The listing builds one solid part. Answer for the finished solid, in the listing's coordinates (mm). Face numbers are marked on the shaded views. A direction names the side the tool comes from. Give positions to 0.01 mm unless a question says otherwise; leave off trailing zeros. Order: outer loops, then holes, each group sorted by start corner. A loop starts at its lowest first (then second) coordinate and runs counter-clockwise, first axis right, second up. Notation, with made-up numbers: (88, -10.75) - (142, -10.75) arc R26 ccw to (142, 19.25) - close; hole circle Ø10 at (51, 22). An arc over 180 degrees is marked (long way). Answer in a Markdown table with one row per item. Add a question column.
```python
from build123d import *

# Parameters (mm, degrees)
PAD027_DEPTH    = 40
PAD028_DEPTH    = 52.4
SKETCH048_W     = 90.6
SKETCH048_H     = 42.3
PAD029_DEPTH    = 1
SKETCH049_R     = 38
POCKET015_DEPTH = 1
POCKET016_DEPTH = 46.3
SKETCH051_R     = 2.15
POCKET017_DEPTH = 1
SKETCH063_W     = 90.6
SKETCH063_H     = 1
PAD033_DEPTH    = 18
SKETCH069_R     = 3.25
POCKET028_DEPTH = 1
SKETCH071_W     = 4
SKETCH071_H     = 6
POCKET030_DEPTH = 1


with BuildPart() as part:
    # Sketch047 → Pad027 (new body)
    with BuildSketch(Plane.XZ):
        Polygon((-45.3, 42), (-46.3, 42), (-46.3, 85.3), (46.3, 85.3), (46.3, 42), (45.3, 42), (45.3, 84.3), (-45.3, 84.3), align=None)
    extrude(amount=PAD027_DEPTH)

    # Sketch047 → Pad028 (join)
    with BuildSketch(Plane.XZ):
        Polygon((-45.3, 42), (-46.3, 42), (-46.3, 85.3), (46.3, 85.3), (46.3, 42), (45.3, 42), (45.3, 84.3), (-45.3, 84.3), align=None)
    extrude(amount=-PAD028_DEPTH)

    # Sketch048 → Pad029 (join)
    with BuildSketch(Plane.XZ):
        with Locations((0, 63.15)):
            Rectangle(SKETCH048_W, SKETCH048_H)
    extrude(amount=PAD029_DEPTH)

    # Sketch049 → Pocket015 (cut)
    with BuildSketch(Plane.XZ):
        with Locations((0, 43)):
            Circle(SKETCH049_R)
    extrude(amount=POCKET015_DEPTH, mode=Mode.SUBTRACT)

    # Sketch050 → Pocket016 (cut, symmetric)
    with BuildSketch(Plane.YZ):
        Polygon((-5, 42), (-40, 84.3), (-40, 42), align=None)
    extrude(amount=POCKET016_DEPTH, both=True, mode=Mode.SUBTRACT)

    # Sketch051 → Pocket017 (cut)
    with BuildSketch(Plane.XZ):
        with Locations((-35.75, 78.75)):
            Circle(SKETCH051_R)
        with Locations((35.75, 78.75)):
            Circle(SKETCH051_R)
    extrude(amount=POCKET017_DEPTH, mode=Mode.SUBTRACT)

    # Sketch063 (on Face12 of Pocket017) → Pad033 (join)
    with BuildSketch(Plane(origin=(0, 0, 84.3), x_dir=(1, 0, 0), z_dir=(0, 0, -1))):
        with Locations((0, 22.5)):
            Rectangle(SKETCH063_W, SKETCH063_H)
    extrude(amount=PAD033_DEPTH)

    # Sketch069 (on Face13 of Pad033) → Pocket028 (cut)
    with BuildSketch(Plane.XZ.offset(23)):
        with Locations((-35.75, 78.75)):
            Circle(SKETCH069_R)
        with Locations((35.75, 78.75)):
            Circle(SKETCH069_R)
    extrude(amount=-POCKET028_DEPTH, mode=Mode.SUBTRACT)

    # Sketch071 → Pocket030 (cut)
    with BuildSketch(Plane.XZ):
        with Locations((43.3, 81.3)):
            Rectangle(SKETCH071_W, SKETCH071_H)
    extrude(amount=POCKET030_DEPTH, mode=Mode.SUBTRACT)


solid = part.part
```
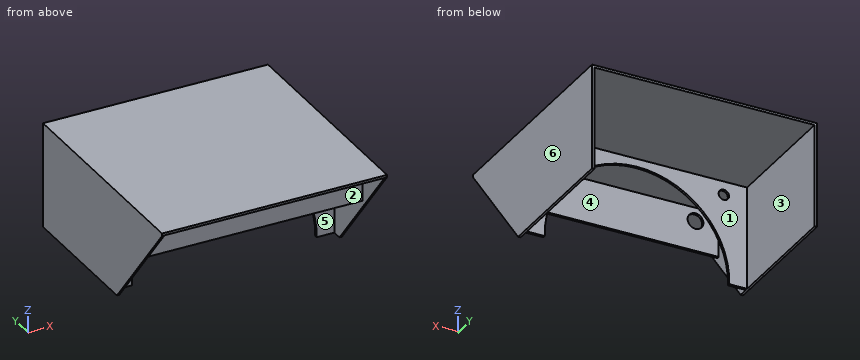
(1) For the marked faces 5 and 6, determine the directions among +Z, -Z, +X, -X, +Y, -Y from which every point of the face is accessible in a straight line to the end or side of a thin tool.
(2) Find section A-A, the plane x = 0. Write down the section's boundary in (y, z), plus the area to 3 significant figures.
(3) Find section B-B, the plane z = 46. Write down the section's boundary in (x, y).
(4) The mould has two halves that part along Y. Classify the marked faces 1, 2, 3 and 4: +Y half, -Y half, draft (parallel to the pull), parting line (faces both ways), or undercut.
(5) Each of these flat-tipped pins is pushed along its axis until it touches: P1, Ø22.5, axis at x = -6, y = 2, coming from the -Z side; P2, Ø12.5, axis at x = 11.5, z = 61, coming from the -Y side; P3, Ø0.5, axis at x = 22, y = -22.5, coming from the -Z side. Where does it stop, or does it pass through?
(6) Find section C-C, the plane x = 35.75. Write down the section's boundary in (y, z), plus the area to 3 significant figures.
(7) Find section D-D, the plane y = 37.5. Write down the section's boundary in (x, z).
(8) Straight lines are drawn through the part: line 1 (Y direction, x = 10, z = 83.5); line 2 (X direction, y = 21, z = 66.5); line 3 (Z direction, x = -35.75, y = -22.75). For each, find the intervals that lie inside material, in ascending order.
Answer key:
| question | item | result |
|---|---|---|
| 1 | face 5 | -Z |
| 1 | face 6 | +Z, -Z, +X, +Y, -Y |
| 2 | outline | (-40, 84.3) - (-23, 84.3) - (-23, 66.3) - (-22, 66.3) - (-22, 84.3) - (-1, 84.3) - (-1, 81) - (0, 81) - (0, 84.3) - (52.4, 84.3) - (52.4, 85.3) - (-40, 85.3) - close |
| 2 | area | 114 mm² |
| 3 | outline | (-46.3, -8.31) - (-45.3, -8.31) - (-45.3, -1) - (-37.88, -1) - (-37.88, 0) - (-45.3, 0) - (-45.3, 52.4) - (-46.3, 52.4) - close; (37.88, -1) - (45.3, -1) - (45.3, -8.31) - (46.3, -8.31) - (46.3, 52.4) - (45.3, 52.4) - (45.3, 0) - (37.88, 0) - close |
| 4 | face 1 | +Y half |
| 4 | face 2 | -Y half |
| 4 | face 3 | draft |
| 4 | face 4 | undercut |
| 5 | P1 | z = 76.95 |
| 5 | P2 | y = -23 |
| 5 | P3 | z = 66.3 |
| 6 | outline | (-40, 84.3) - (-23, 84.3) - (-23, 82) - (-22, 82) - (-22, 84.3) - (-1, 84.3) - (-1, 80.9) - (0, 80.9) - (0, 84.3) - (52.4, 84.3) - (52.4, 85.3) - (-40, 85.3) - close; (-23, 66.3) - (-22, 66.3) - (-22, 75.5) - (-23, 75.5) - close; (-1, 55.88) - (0, 55.88) - (0, 76.6) - (-1, 76.6) - close |
| 6 | area | 128 mm² |
| 7 | outline | (-46.3, 42) - (-45.3, 42) - (-45.3, 84.3) - (45.3, 84.3) - (45.3, 42) - (46.3, 42) - (46.3, 85.3) - (-46.3, 85.3) - close |
| 8 | line 1 | -23 to -22, -1 to 0 |
| 8 | line 2 | -46.3 to -45.3, 45.3 to 46.3 |
| 8 | line 3 | 66.3 to 75.5, 82 to 85.3 |
